```python
from build123d import *

# Parameters (mm, degrees)
BOSS_EXTRUDE1_DEPTH = 15.5
FILLET1_R           = 7
FILLET2_R           = 10
FILLET3_R           = 5
FILLET4_R           = 2
SKETCH2_R           = 1.5
SKETCH2_W           = 10.92280205
SKETCH2_H           = 2.497802755
SKETCH2_W_2         = 14.300247421
SKETCH2_H_2         = 2.745251167
SKETCH2_W_3         = 6.180006424
SKETCH2_H_3         = 2.556024723
SKETCH2_W_4         = 7.044858218
SKETCH2_W_5         = 10.276057193
SKETCH2_H_4         = 2.946282132
SKETCH2_W_6         = 7.976519918
SKETCH2_W_7         = 7.689077759
SKETCH2_W_8         = 8.982567476
SKETCH2_H_5         = 2.60403982
SKETCH2_W_9         = 6.180006423
SKETCH2_W_10        = 10.172310113
SKETCH2_H_6         = 2.663918404
SKETCH2_W_11        = 5.94485656
SKETCH2_H_7         = 2.427407937
SKETCH2_W_12        = 5.086155057
SKETCH2_H_8         = 2.229246052
SKETCH2_H_9         = 2.744285017
SKETCH2_W_13        = 9.577824458
CUT_EXTRUDE1_DEPTH  = 3.5


with BuildPart() as part:
    # Sketch1 → Boss-Extrude1 (new body)
    with BuildSketch(Plane(origin=(0, 0, 0), x_dir=(1, 0, 0), z_dir=(0, 1, 0))):
        Polygon((25, -40.75), (-25, -40.75), (-25, -20.75), (-20, -20.75), (-20, 25.75), (-25, 25.75), (-25, 40.75), (25, 40.75), (25, 25.75), (20, 25.75), (20, -20.75), (25, -20.75), align=None)
    extrude(amount=BOSS_EXTRUDE1_DEPTH)

    # Fillet1
    fillet1_edges = [part.edges().sort_by_distance(p)[0] for p in [
        (-25, 7.75, -40.75),
        (25, 7.75, -40.75),
        (25, 7.75, 40.75),
        (-25, 7.75, 40.75),
    ]]
    fillet(fillet1_edges, radius=FILLET1_R)

    # Fillet2
    # the kernel refuses this fillet: 10 mm, written as the material it adds along each edge
    with BuildSketch(Plane(origin=(-20, 0, 20.75), x_dir=(-1, 0, 0), z_dir=(0, 1, 0))) as fillet2_piece_1:
        with BuildLine():
            CenterArc((10, -8.660254038), FILLET2_R, 120, 60)
            Line((0, -8.660254038), (-0.2, -8.660254038))
            Line((-0.2, -8.660254038), (-0.2, 0))
            Line((-0.2, 0), (0, 0.2))
            ThreePointArc((0, 0.2), (2.5, 0.2), (4.9, 0.173205081))
            Line((4.9, 0.173205081), (5, 0))
        make_face()
    extrude(amount=15.5)
    with BuildSketch(Plane(origin=(-20, 0, -25.75), x_dir=(0, 0, 1), z_dir=(0, 1, 0))) as fillet2_piece_2:
        with BuildLine():
            CenterArc((8.660254038, -10), FILLET2_R, 90, 60)
            Line((0, -5), (-0.173205081, -4.9))
            ThreePointArc((-0.173205081, -4.9), (-0.2, -2.5), (-0.2, 0))
            Line((-0.2, 0), (0, 0.2))
            Line((0, 0.2), (8.660254038, 0.2))
            Line((8.660254038, 0.2), (8.660254038, 0))
        make_face()
    extrude(amount=15.5)
    with BuildSketch(Plane(origin=(20, 0, 20.75), x_dir=(1, 0, 0), z_dir=(0, 1, 0))) as fillet2_piece_3:
        with BuildLine():
            CenterArc((10, 8.660254038), FILLET2_R, 180, 60)
            Line((0, 8.660254038), (-0.2, 8.660254038))
            Line((-0.2, 8.660254038), (-0.2, 0))
            Line((-0.2, 0), (0, -0.2))
            ThreePointArc((0, -0.2), (2.5, -0.2), (4.9, -0.173205081))
            Line((4.9, -0.173205081), (5, 0))
        make_face()
    extrude(amount=15.5)
    with BuildSketch(Plane(origin=(20, 0, -25.75), x_dir=(0, 0, 1), z_dir=(0, 1, 0))) as fillet2_piece_4:
        with BuildLine():
            CenterArc((8.660254038, 10), FILLET2_R, 210, 60)
            Line((0, 5), (-0.173205081, 4.9))
            ThreePointArc((-0.173205081, 4.9), (-0.2, 2.5), (-0.2, 0))
            Line((-0.2, 0), (0, -0.2))
            Line((0, -0.2), (8.660254038, -0.2))
            Line((8.660254038, -0.2), (8.660254038, 0))
        make_face()
    extrude(amount=15.5)

    # Fillet3
    fillet3_edges = [part.edges().sort_by_distance(p)[0] for p in [
        (25, 7.75, -25.75),
        (25, 7.75, 20.75),
        (-25, 7.75, 20.75),
        (-25, 7.75, -25.75),
    ]]
    fillet(fillet3_edges, radius=FILLET3_R)

    # Fillet4
    fillet4_edges = [part.edges().sort_by_distance(p)[0] for p in [
        (0, 0, -40.75),
        (0, 15.5, -40.75),
        (-25, 0, -31.010042925),
        (25, 0, 28.510042925),
        (0, 0, 40.75),
        (22.949747468, 0, 38.699747468),
        (-22.949747468, 0, 38.699747468),
        (-22.949747468, 0, -38.699747468),
        (22.949747468, 0, -38.699747468),
        (-25, 15.5, -31.010042925),
        (0, 15.5, 40.75),
        (25, 15.5, 28.510042925),
        (22.949747468, 15.5, 38.699747468),
        (-22.949747468, 15.5, 38.699747468),
        (-22.949747468, 15.5, -38.699747468),
        (22.949747468, 15.5, -38.699747468),
        (-20, 0, -2.5),
        (-20, 15.5, -2.5),
        (20, 0, -2.5),
        (20, 15.5, -2.5),
        (-20.871290708, 15.5, 16.172228867),
        (-20.871290708, 0, -21.172228867),
        (20.871290708, 0, 16.172228867),
        (20.871290708, 15.5, -21.172228867),
        (-25, 0, 28.510042925),
        (-25, 15.5, 28.510042925),
        (25, 0, -31.010042925),
        (20.871290708, 0, -21.172228867),
        (-20.871290708, 0, 16.172228867),
        (-24.564354646, 0, -26.228844397),
        (24.564354646, 0, -26.228844397),
        (24.564354646, 0, 21.228844397),
        (-24.564354646, 0, 21.228844397),
        (25, 15.5, -31.010042925),
        (-20.871290708, 15.5, -21.172228867),
        (20.871290708, 15.5, 16.172228867),
        (-24.564354646, 15.5, -26.228844397),
        (24.564354646, 15.5, -26.228844397),
        (24.564354646, 15.5, 21.228844397),
        (-24.564354646, 15.5, 21.228844397),
    ]]
    fillet(fillet4_edges, radius=FILLET4_R)

    # Sketch2 → Cut-Extrude1 (cut)
    with BuildSketch(Plane(origin=(0, 15.5, 0), x_dir=(1, 0, 0), z_dir=(0, 1, 0))):
        with Locations(Location((-21.439879839, -29.907193015, 0), (0, 0, 270))):
            Circle(SKETCH2_R)
        with Locations(Location((21.392609924, -29.907193015, 0), (0, 0, 270))):
            Circle(SKETCH2_R)
        with Locations(Location((-19.83836984, 31.824604268, 0), (0, 0, 270))):
            Circle(SKETCH2_R)
        with Locations(Location((19.72370758, 31.824604268, 0), (0, 0, 270))):
            Circle(SKETCH2_R)
        with Locations((-13.747194041, -35.095106184)):
            Rectangle(SKETCH2_W, SKETCH2_H)
        with Locations((-12.058471356, -25.845093422)):
            Rectangle(SKETCH2_W_2, SKETCH2_H_2)
        with Locations((16.290511598, -35.0659952)):
            Rectangle(SKETCH2_W_3, SKETCH2_H_3)
        with Locations((16.72604395, -25.845093422)):
            Rectangle(SKETCH2_W_4, SKETCH2_H_2)
        with Locations((-12.000710148, -16.003419816)):
            Rectangle(SKETCH2_W_5, SKETCH2_H_4)
        with Locations((0, -16.003419816)):
            Rectangle(SKETCH2_W_6, SKETCH2_H_4)
        with Locations((12.791176086, -16.003419816)):
            Rectangle(SKETCH2_W_7, SKETCH2_H_4)
        with Locations((-12.647455006, 1.143849121)):
            Rectangle(SKETCH2_W_8, SKETCH2_H_5)
        with Locations((-0.251511889, 1.143849121)):
            Rectangle(SKETCH2_W_9, SKETCH2_H_5)
        with Locations((12.008853949, 1.173788413)):
            Rectangle(SKETCH2_W_10, SKETCH2_H_6)
        with Locations((-6.750471196, 7.68245568)):
            Rectangle(SKETCH2_W_11, SKETCH2_H_7)
        with Locations((6.361240217, 7.583374737)):
            Rectangle(SKETCH2_W_12, SKETCH2_H_8)
        with Locations((-12.647455006, -7.655884762)):
            Rectangle(SKETCH2_W_8, SKETCH2_H_9)
        with Locations((12.4382047, -7.655884762)):
            Rectangle(SKETCH2_W_13, SKETCH2_H_9)
    extrude(amount=-CUT_EXTRUDE1_DEPTH, mode=Mode.SUBTRACT)


solid = part.part
```
Verification items for the finished model (mm, model axes). A direction names the side the tool comes from. Round coordinates to 2 decimals unless told otherwise and drop trailing zeros. Loops run counter-clockwise (first coordinate to the right, second up) from the corner with the lowest first, then second, coordinate; pieces in that order, holes last. Notation, with made-up numbers: (88.25, -23) -> (97.25, -23) arc R15 cw to (97.25, -3) -> close; hole circle Ø5 at (-30, -25.75). An arc over 180 degrees is marked (long way). Answer as a JSON object with one key per item and string values.
Q1. Section check A-A (y = 9). Record the boundary of the cut face in (x, z).
Data:
{"outline": "(-25, -33.75) arc R7 ccw to (-18, -40.75) -> (18, -40.75) arc R7 ccw to (25, -33.75) -> (25, -28.27) arc R5 ccw to (23.33, -24.54) arc R10 cw to (20, -17.09) -> (20, 12.09) arc R10 cw to (23.33, 19.54) arc R5 ccw to (25, 23.27) -> (25, 33.75) arc R7 ccw to (18, 40.75) -> (-18, 40.75) arc R7 ccw to (-25, 33.75) -> (-25, 23.27) arc R5 ccw to (-23.33, 19.54) arc R10 cw to (-20, 12.09) -> (-20, -17.09) arc R10 cw to (-23.33, -24.54) arc R5 ccw to (-25, -28.27) -> close"}
Q2. Section check B-B (x = -11). Record the boundary of the cut face in (y, z).
Data:
{"outline": "(0, -38.75) arc R2 ccw to (2, -40.75) -> (13.5, -40.75) arc R2 ccw to (15.5, -38.75) -> (15.5, -2.45) -> (12, -2.45) -> (12, 0.16) -> (15.5, 0.16) -> (15.5, 6.28) -> (12, 6.28) -> (12, 9.03) -> (15.5, 9.03) -> (15.5, 14.53) -> (12, 14.53) -> (12, 17.48) -> (15.5, 17.48) -> (15.5, 24.47) -> (12, 24.47) -> (12, 27.22) -> (15.5, 27.22) -> (15.5, 33.85) -> (12, 33.85) -> (12, 36.34) -> (15.5, 36.34) -> (15.5, 38.75) arc R2 ccw to (13.5, 40.75) -> (2, 40.75) arc R2 ccw to (0, 38.75) -> close"}
Q3. Section check C-C (z = 10). Record the boundary of the cut face in (x, y).
Data:
{"outline": "(-20, 2) arc R2 ccw to (-18, 0) -> (18, 0) arc R2 ccw to (20, 2) -> (20, 13.5) arc R2 ccw to (18, 15.5) -> (-18, 15.5) arc R2 ccw to (-20, 13.5) -> close"}
Q4. Go/stop test with flat-tipped pins: P1, Ø1.2, axis at y = 13.5, z = -7, coming from the -X side; P2, Ø0.9, axis at x = 13.5, z = 16.5, coming from the +Y side; P3, Ø1.5, axis at y = 7, z = -21, coming from the -X side. Record where each tip stops, or that it passes through.
Data:
{"P1": "stops at x = -20", "P2": "stops at y = 12", "P3": "stops at x = -21.15"}
Q5. Scan lines: line 1 (Z direction, x = -17.5, y = 12.5); line 2 (X direction, y = 10.75, z = -10.5); line 3 (X direction, y = 2.25, z = -34). Record each from-to range of solid material in increasing order. Write a range as from..to.
Data:
{"line 1": "z = -40.75..24.47, 27.22..33.85, 36.34..40.75", "line 2": "x = -20..20", "line 3": "x = -25..25"}
Q6. Draft check along Z on faces 4 (the cylindrical face through (-24.4, 0.57, -31.05)), 5 (the cylindrical face through (-23, 7.83, -38.65)), 6 (the flat face through (20.248, 14, 26)), 7 (the flat face through (13.201, 14, 35)). Enter one of: pulls with the +Z half, pulls with the -Z half, needs draft (parallel to the pull), parting line crosses it, or undercut.
Data:
{"face 4": "needs draft", "face 5": "pulls with the -Z half", "face 6": "undercut", "face 7": "undercut"}
Q7. Section check D-D (x = 14.5). Record the boundary of the cut face in (y, z).
Data:
{"outline": "(0, -38.75) arc R2 ccw to (2, -40.75) -> (13.5, -40.75) arc R2 ccw to (15.5, -38.75) -> (15.5, -2.51) -> (12, -2.51) -> (12, 0.16) -> (15.5, 0.16) -> (15.5, 6.28) -> (12, 6.28) -> (12, 9.03) -> (15.5, 9.03) -> (15.5, 14.53) -> (12, 14.53) -> (12, 17.48) -> (15.5, 17.48) -> (15.5, 24.47) -> (12, 24.47) -> (12, 27.22) -> (15.5, 27.22) -> (15.5, 33.79) -> (12, 33.79) -> (12, 36.34) -> (15.5, 36.34) -> (15.5, 38.75) arc R2 ccw to (13.5, 40.75) -> (2, 40.75) arc R2 ccw to (0, 38.75) -> close"}
Q8. Access from +Z, -Z, +X, -X, +Y, -Y to the whole of each face (thin tool, end or side, straight path). Record for faces 1 (the flat face through (-21, 12, 30)), 2 (the flat face through (25, 8, 28)), 3 (the cylindrical face through (20.85, 7.67, 16.12)).
Data:
{"face 1": "+Y", "face 2": "+Z, -Z, +X, +Y, -Y", "face 3": "+X, +Y, -Y"}
